Model file for the job. Use its own axes, mm. A direction names the side the tool comes from. Round coordinates to 2 decimals unless told otherwise and drop trailing zeros. Order: outer loops, then holes, each group sorted by start corner. A loop starts at its lowest first (then second) coordinate and runs counter-clockwise, first axis right, second up. Notation, with made-up numbers: (16.5, 86) -> (44.5, 86) arc R15 cw to (44.5, 95) -> close; hole circle Ø6 at (54.5, 55). An arc over 180 degrees is marked (long way). Answer as CSV lines item,"result".
```python
from build123d import *

# Parameters (mm, degrees)
F0_W     = 10.2
F0_H     = 70
F1_DEPTH = 15
F2_SIZE  = 1


with BuildPart() as f1:
    # F0 (on Top) → F1 (new body)
    with BuildSketch(Plane.XY):
        Polygon((20, 0), (0, 0), (-20, 0), (-20, -80), (0, -80), (20, -80), align=None)
        with Locations((-7.3, -40)):
            Rectangle(F0_W, F0_H, mode=Mode.SUBTRACT)
        with Locations((7.3, -40)):
            Rectangle(F0_W, F0_H, mode=Mode.SUBTRACT)
    extrude(amount=F1_DEPTH)

    # F2
    f2_edges = [f1.edges().sort_by_distance(p)[0] for p in [
        (0, 0, 15),
        (-20, -40, 15),
        (0, -80, 15),
        (20, -40, 15),
        (-7.3, -75, 15),
        (-12.4, -40, 15),
        (-7.3, -5, 15),
        (-2.2, -40, 15),
        (7.3, -5, 15),
        (12.4, -40, 15),
        (7.3, -75, 15),
        (2.2, -40, 15),
    ]]
    chamfer(f2_edges, length=F2_SIZE)


solid = f1.part
```
Q1. Saw through at B-B (x = -11.5). Write the cut outline in (y, z).
Checks:
outline,"(-80, 0) -> (-75, 0) -> (-75, 14) -> (-76, 15) -> (-79, 15) -> (-80, 14) -> close; (-5, 0) -> (0, 0) -> (0, 14) -> (-1, 15) -> (-4, 15) -> (-5, 14) -> close"
Q2. Saw through at A-A (y = -21). Write the cut outline in (x, z), plus the area to 3 significant figures.
Checks:
outline,"(-20, 0) -> (-12.4, 0) -> (-12.4, 14) -> (-13.4, 15) -> (-19, 15) -> (-20, 14) -> close; (-2.2, 0) -> (2.2, 0) -> (2.2, 14) -> (1.2, 15) -> (-1.2, 15) -> (-2.2, 14) -> close; (12.4, 0) -> (20, 0) -> (20, 14) -> (19, 15) -> (13.4, 15) -> (12.4, 14) -> close"
area,"291 mm²"
Q3. Mould opens along Y. For faces 3 (the flat face through (0, 0, 7)), 4 (the flat face through (12.4, -40, 7)), 5 (the flat face through (0, -37, 15)) say: +Y half, -Y half, draft (parallel to the pull), parting line (faces both ways), or undercut.
Checks:
face 3,"+Y half"
face 4,"undercut"
face 5,"draft"
Q4. Wall check: L1, parallel to X at y = -48, z = 9.25; L2, parallel to Y at x = 3, z = 3.25. Give the ranges that are in metal, low to high. Write a range as [from, to].
Checks:
L1,"[-20, -12.4], [-2.2, 2.2], [12.4, 20]"
L2,"[-80, -75], [-5, 0]"
Q5. Saw through at C-C (z = 3.25). Write the cut outline in (x, y).
Checks:
outline,"(-20, -80) -> (20, -80) -> (20, 0) -> (-20, 0) -> close; hole (-12.4, -75) -> (-2.2, -75) -> (-2.2, -5) -> (-12.4, -5) -> close; hole (2.2, -75) -> (12.4, -75) -> (12.4, -5) -> (2.2, -5) -> close"
Q6. Flat gauge pin, fed straight in: pin 1 (4 mm diameter, centred on x = -10.5, y = -10, fed in from +Z). Where does the tip first touch, or does it go through?
Checks:
pin 1,"z = 14.1"
Q7. Tool access for faces 1 (the flat face through (-12.4, -40, 7)), 2 (the flat face through (-20, -39, 7)): list every direction of +Z, -Z, +X, -X, +Y, -Y with a clear straight run to the whole face (end or side of a thin tool).
Checks:
face 1,"+Z, -Z"
face 2,"+Z, -Z, -X, +Y, -Y"
